Could you check a few things on this model? Use its own coordinates, in mm. A direction names the side the tool comes from. Give positions to 0.01 mm unless a question says otherwise; leave off trailing zeros. Write each loop counter-clockwise with the first axis right and the second up, starting at its lowest first coordinate (ties: lowest second). Pieces come first, ordered by that corner, then holes. Notation, with made-up numbers: M -33.75,46.25 L -1.75,46.25 A22 ccw -1.75,79.25 Z; hole C 76.5,55.25 d8. An arc over 180 degrees is marked long. Use one line per item in the form item = value.
Autodesk Inventor part; units mm, degrees
ref_plane "YZ Plane" through (0, 0, 0) normal (1, 0, 0) x (0, 1, 0)
ref_plane "XZ Plane" through (0, 0, 0) normal (0, 1, 0) x (-1, 0, 0)
ref_plane "XY Plane" through (0, 0, 0) normal (0, 0, 1) x (1, 0, 0)
sketch "Sketch1" plane through (0, 0, 0) normal (1, 0, 0) x (0, 1, 0)
  line L0 (0, 0) -> (-210, 0)
  line L1 (-210, 0) -> (-210, -300)
  line L2 (-210, -300) -> (0, -300)
  line L3 (0, -300) -> (0, 0)
  dimension "d0" = 210
  dimension "d1" = 300
extrude "Extrusion1" add sketch "Sketch1" along normal blind 101.6
sketch "Sketch2" plane through (101.6, 0, 0) normal (1, 0, 0) x (0, 0, -1)
  line L0 (0, -210) -> (300, -210)
  line L1 (300, -210) -> (300, 0)
  line L2 (300, 0) -> (0, 0)
  line L3 (0, 0) -> (0, -210)
  line L4 (1.6, -1.6) -> (298.4, -1.6)
  line L5 (298.4, -1.6) -> (298.4, -208.4)
  line L6 (298.4, -208.4) -> (1.6, -208.4)
  line L7 (1.6, -208.4) -> (1.6, -1.6)
  dimension "d4" = 1.6
extrude "Extrusion2" cut sketch "Sketch2" against normal blind 100 contours L4 L5 L6 L7
sketch "Sketch3" plane through (1.6, 0, 0) normal (1, 0, 0) x (0, 0, -1)
  circle A0 centre (75.3333, -47.4667) radius 4
  circle A1 centre (215.3333, -47.4667) radius 4
  circle A2 centre (215.3333, -158.4667) radius 4
  circle A3 centre (75.3333, -158.4667) radius 4
  point P0 (0, 0)
  dimension "d7" = 8
  dimension "d8" = 8
  dimension "d9" = 8
  dimension "d10" = 8
  dimension "d11" = 140
  dimension "d12" = 111
extrude "Extrusion3" add sketch "Sketch3" along normal blind 12
sketch "Sketch4" plane through (13.6, -47.4667, -75.3333) normal (1, 0, 0) x (0, 0, -1)
  circle A0 centre (0, 0) radius 4
  circle A1 centre (140, 0) radius 4
  circle A2 centre (140, -111) radius 4
  circle A3 centre (0, -111) radius 4
  point P0 (-75.3333, 47.4667)
hole "Hole1" at (13.6, -47.4667, -75.3333) at (13.6, -47.4667, -215.3333) at (13.6, -158.4667, -215.3333) at (13.6, -158.4667, -75.3333) direction (-1, 0, 0) diameter 2.8 depth 10.4
sketch "Sketch5" plane through (101.6, 0, 0) normal (1, 0, 0) x (0, 0, -1)
  line L0 (5.6, -5.6) -> (95.6, -5.6)
  line L1 (95.6, -5.6) -> (95.6, -127.6)
  line L2 (95.6, -127.6) -> (5.6, -127.6)
  line L3 (5.6, -127.6) -> (5.6, -5.6)
  line L4 (1.6, -208.4) -> (1.6, -1.6)
  line L5 (1.6, -1.6) -> (298.4, -1.6)
  line L6 (103.6, -5.6) -> (193.6, -5.6)
  line L7 (103.6, -127.6) -> (103.6, -5.6)
  line L8 (193.6, -5.6) -> (193.6, -127.6)
  line L9 (193.6, -127.6) -> (103.6, -127.6)
  line L10 (201.6, -5.6) -> (291.6, -5.6)
  line L11 (201.6, -127.6) -> (201.6, -5.6)
  line L12 (291.6, -5.6) -> (291.6, -127.6)
  line L13 (291.6, -127.6) -> (201.6, -127.6)
  line L14 (298.4, -1.6) -> (298.4, -208.4)
  line L15 (292.4, -132.4) -> (244.4, -132.4)
  line L16 (244.4, -132.4) -> (244.4, -202.4)
  line L17 (244.4, -202.4) -> (292.4, -202.4)
  line L18 (292.4, -202.4) -> (292.4, -132.4)
  line L19 (298.4, -208.4) -> (1.6, -208.4)
  line L20 (190.4, -132.4) -> (190.4, -202.4)
  line L21 (238.4, -132.4) -> (190.4, -132.4)
  line L22 (238.4, -202.4) -> (238.4, -132.4)
  line L23 (190.4, -202.4) -> (238.4, -202.4)
  line L24 (136.4, -132.4) -> (136.4, -202.4)
  line L25 (184.4, -132.4) -> (136.4, -132.4)
  line L26 (184.4, -202.4) -> (184.4, -132.4)
  line L27 (136.4, -202.4) -> (184.4, -202.4)
  line L28 (82.4, -132.4) -> (82.4, -202.4)
  line L29 (130.4, -132.4) -> (82.4, -132.4)
  line L30 (130.4, -202.4) -> (130.4, -132.4)
  line L31 (82.4, -202.4) -> (130.4, -202.4)
  point P0 (0, 0)
  point P1 (268.4, -202.4)
  point P2 (214.4, -202.4)
  point P3 (160.4, -202.4)
  point P4 (106.4, -202.4)
  dimension "d22" = 90
  dimension "d23" = 122
  dimension "d24" = 4
  dimension "d25" = 4
  dimension "d28" = 98
  dimension "d33" = 6.8
  dimension "d34" = 48
  dimension "d35" = 70
  dimension "d36" = 6
  dimension "d37" = 6
  dimension "d40" = 54
extrude "Extrusion4" add sketch "Sketch5" against normal blind 4
equation "\"d8\" = d7"
equation "\"d9\" = d7"
equation "\"d10\" = d7"
equation "\"d25\" = d24"
equation "\"d37\" = d36"
1) If I drill on L1, parallel to X at y = -10, z = -101.5; L2, parallel to Y at x = 20.5, z = -37.5; L3, parallel to Z at x = 37, y = -36, over which ranges is the centre line in solid material (lowest first)?
Checked values:
L1 = 0 to 1.6, 97.6 to 101.6
L2 = -210 to -208.4, -1.6 to 0
L3 = -300 to -298.4, -1.6 to 0
2) For pin 1 Ø10 at (y, z) = (-96.5, -270) entering from -X; pin 2 Ø2 at (y, z) = (-158, -215) entering from +X; pin 3 Ø4 at (y, z) = (-150, -168) entering from +X; pin 4 Ø1.7 at (y, z) = (-47.47, -215.33) entering from +X, each with a flat end and sliding along its axis, tell me the tip position at first contact or that it passes through.
Checked values:
pin_1 = 0
pin_2 = 13.6
pin_3 = 1.6
pin_4 = 3.2
3) I want a section at A-A, the plane x = 28.5. Please give me the cut outline in (y, z), plus the area to 3 significant figures.
Checked values:
outline = M -210,-300 L 0,-300 L 0,0 L -210,0 Z; hole M -208.4,-298.4 L -1.6,-298.4 L -1.6,-1.6 L -208.4,-1.6 Z
area = 1,620 mm2
4) I want a section at B-B, the plane z = -180.5. Please give me the cut outline in (x, y), plus the area to 3 significant figures.
Checked values:
outline = M 0,-210 L 101.6,-210 L 101.6,-202.4 L 97.6,-202.4 L 97.6,-208.4 L 1.6,-208.4 L 1.6,-1.6 L 97.6,-1.6 L 97.6,-5.6 L 101.6,-5.6 L 101.6,0 L 0,0 Z; M 97.6,-132.4 L 101.6,-132.4 L 101.6,-127.6 L 97.6,-127.6 Z
area = 715 mm2
5) Thinking about a two-plate mould opening in X: for faces 1 (the flat face through (50, -210, -148)), 2 (the flat face through (101.6, -128, -127)), 3 (the flat face through (50, -1.6, -148)), which applies, released by +X, released by -X, zero draft, split by the parting line, or undercut?
Checked values:
face_1 = zero draft
face_2 = released by +X
face_3 = undercut
6) I want a section at D-D, the plane z = -48.5. Please give me the cut outline in (x, y).
Checked values:
outline = M 0,-210 L 101.6,-210 L 101.6,-127.6 L 97.6,-127.6 L 97.6,-208.4 L 1.6,-208.4 L 1.6,-1.6 L 97.6,-1.6 L 97.6,-5.6 L 101.6,-5.6 L 101.6,0 L 0,0 Z
7) I want a section at C-C, the plane y = -124.5. Please give me the cut outline in (x, z).
Checked values:
outline = M 0,-300 L 101.6,-300 L 101.6,-291.6 L 97.6,-291.6 L 97.6,-298.4 L 1.6,-298.4 L 1.6,-1.6 L 97.6,-1.6 L 97.6,-5.6 L 101.6,-5.6 L 101.6,0 L 0,0 Z; M 97.6,-201.6 L 101.6,-201.6 L 101.6,-193.6 L 97.6,-193.6 Z; M 97.6,-103.6 L 101.6,-103.6 L 101.6,-95.6 L 97.6,-95.6 Z
8) For faces 4 (the flat face through (50, -106, -300)), 5 (the cylindrical face through (7.52, -154.56, -74.47)), 6 (the cylindrical face through (7.52, -154.56, -214.47)), which set-ups out of +Z, -Z, +X, -X, +Y, -Y let a thin tool reach every point of the face, with its end or its side?
Checked values:
face_4 = -Z, +X, -X, +Y, -Y
face_5 = none
face_6 = +X
